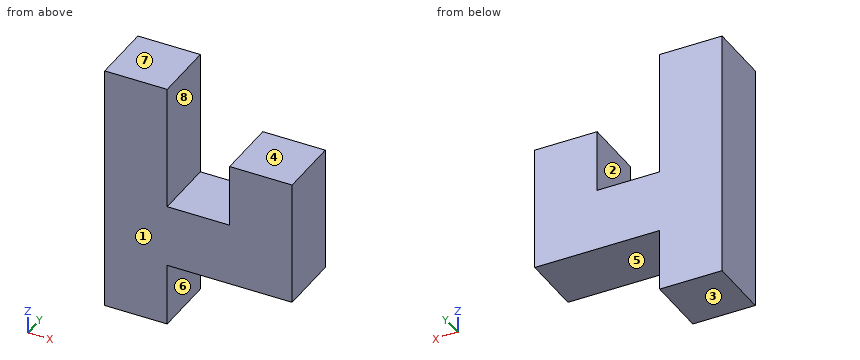
from build123d import *

# Parameters (mm, degrees)
F0_W     = 12.7
F0_H     = 12.7
F1_DEPTH = 6.35


with BuildPart() as f1:
    # F0 (on Front) → F1 (new body, symmetric)
    with BuildSketch(Plane.XZ):
        with Locations((-49.254278, 46.948222)):
            Rectangle(F0_W, F0_H)
        with Locations((-49.254278, 34.248222)):
            Rectangle(F0_W, F0_H)
        with Locations((-49.254278, 21.548222)):
            Rectangle(F0_W, F0_H)
        with Locations((-36.554278, 21.548222)):
            Rectangle(F0_W, F0_H)
        with Locations((-49.254278, 8.848222)):
            Rectangle(F0_W, F0_H)
        with Locations((-23.854278, 21.548222)):
            Rectangle(F0_W, F0_H)
        with Locations((-23.854278, 34.248222)):
            Rectangle(F0_W, F0_H)
    extrude(amount=F1_DEPTH, both=True)


solid = f1.part
Could you check a few things on this model? Use its own coordinates, in mm. Face numbers are marked on the shaded views. A direction names the side the tool comes from. Round coordinates to 2 decimals unless told otherwise and drop trailing zeros. Write each loop counter-clockwise with the first axis right and the second up, starting at its lowest first coordinate (ties: lowest second). Pieces come first, ordered by that corner, then holes. Notation, with made-up numbers: (28.5, 89.5) - (59.5, 89.5) arc R21 cw to (59.5, 112.5) - close; hole circle Ø4 at (-19.75, 69). An arc over 180 degrees is marked (long way). Use a Markdown table: item, result.
Q1. I want a section at A-A (z = 34). List the corners of the cut face in (x, y) for me, plus the area to 3 significant figures.
Output values:
| item | result |
|---|---|
| outline | (-55.6, -6.35) - (-42.9, -6.35) - (-42.9, 6.35) - (-55.6, 6.35) - close; (-30.2, -6.35) - (-17.5, -6.35) - (-17.5, 6.35) - (-30.2, 6.35) - close |
| area | 323 mm2 |
Q2. I want a section at D-D (z = 12). List the corners of the cut face in (x, y) for me, plus the area to 3 significant figures.
Output values:
| item | result |
|---|---|
| outline | (-55.6, -6.35) - (-42.9, -6.35) - (-42.9, 6.35) - (-55.6, 6.35) - close |
| area | 161 mm2 |
Q3. I want a section at B-B (y = -1). List the corners of the cut face in (x, z) for me.
Output values:
| item | result |
|---|---|
| outline | (-55.6, 2.5) - (-42.9, 2.5) - (-42.9, 15.2) - (-17.5, 15.2) - (-17.5, 40.6) - (-30.2, 40.6) - (-30.2, 27.9) - (-42.9, 27.9) - (-42.9, 53.3) - (-55.6, 53.3) - close |
Q4. I want a section at C-C (x = -35). List the corners of the cut face in (y, z) for me.
Output values:
| item | result |
|---|---|
| outline | (-6.35, 15.2) - (6.35, 15.2) - (6.35, 27.9) - (-6.35, 27.9) - close |
Q5. For the marked faces 1, 2, 3, 4 and 5, which set-ups out of +Z, -Z, +X, -X, +Y, -Y let a thin tool reach every point of the face, with its end or its side?
Output values:
| item | result |
|---|---|
| face 1 | +Z, -Z, +X, -X, -Y |
| face 2 | +Z, +Y, -Y |
| face 3 | -Z, +X, -X, +Y, -Y |
| face 4 | +Z, +X, +Y, -Y |
| face 5 | -Z, +X, +Y, -Y |
Q6. For pin 1 (6 mm diameter, centred on x = -28, y = 1, fed in from -Z); pin 2 (1.5 mm diameter, centred on y = -2.5, z = 44.5, fed in from +X); pin 3 (5 mm diameter, centred on x = -42, y = 1, fed in from +Z); pin 4 (6.5 mm diameter, centred on x = -26, y = -2.5, fed in from +Z), each with a flat end and sliding along its axis, tell me the tip position at first contact or that it passes through.
Output values:
| item | result |
|---|---|
| pin 1 | z = 15.2 |
| pin 2 | x = -42.9 |
| pin 3 | z = 53.3 |
| pin 4 | z = 40.6 |
Q7. Thinking about a two-plate mould opening in X: for the marked faces 6, 7 and 8, which applies, released by +X, released by -X, zero draft, split by the parting line, or undercut?
Output values:
| item | result |
|---|---|
| face 6 | released by +X |
| face 7 | zero draft |
| face 8 | undercut |
Q8. Please list where these lines run through material, in increasing order: L1, parallel to X at y = 0, z = 28; L2, parallel to Z at x = -23.5, y = -0.5; L3, parallel to X at y = 5.25, z = 43.
Output values:
| item | result |
|---|---|
| L1 | -55.6 to -42.9, -30.2 to -17.5 |
| L2 | 15.2 to 40.6 |
| L3 | -55.6 to -42.9 |
